Geometry: final body of the model. Coordinates: model frame, mm. Face numbers are marked on the shaded views. Round coordinates to 2 decimals unless told otherwise and drop trailing zeros. Loops run counter-clockwise (first coordinate to the right, second up) from the corner with the lowest first, then second, coordinate; pieces in that order, holes last. Notation, with made-up numbers: (-15.75, -9) -> (33.25, -9) arc R16 cw to (33.25, -5) -> close; hole circle Ø10 at (15.5, 9). An arc over 180 degrees is marked (long way). Answer in a Markdown table with one row per item.
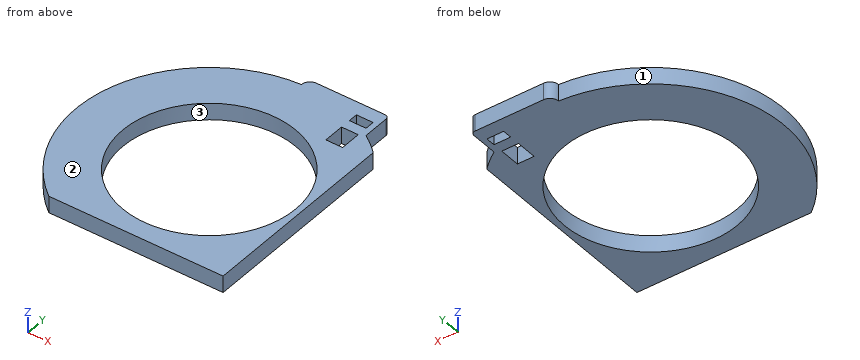
```python
from build123d import *

# Parameters (mm, degrees)
SKETCH1_R           = 25.869040911
BOSS_EXTRUDE1_DEPTH = 5
CUT_EXTRUDE1_REACH  = 7
SKETCH2_W           = 5
SKETCH2_H           = 2.807032228
SKETCH2_H_2         = 6.272905991


with BuildPart() as part:
    # Sketch1 → Boss-Extrude1 (new body)
    with BuildSketch(Plane.XY):
        with BuildLine():
            Line((27.585503877, -31.392941885), (-24.576892053, -31.392941885))
            ThreePointArc((-24.576892053, -31.392941885), (-38.026656197, 11.979726275), (-2.145068244, 39.811293691))
            ThreePointArc((-2.145068244, 39.811293691), (-1.391692185, 41.630104391), (0.427118514, 42.38348045))
            Line((0.427118514, 42.38348045), (20.910674351, 42.38348045))
            ThreePointArc((20.910674351, 42.38348045), (21.815017729, 42.008889157), (22.189609022, 41.104545778))
            Line((22.189609022, 41.104545778), (22.189609022, 33.1234309))
            ThreePointArc((22.189609022, 33.1234309), (24.981909543, 31.071604702), (27.585503877, 28.785072503))
            Line((27.585503877, 28.785072503), (27.585503877, -31.392941885))
        make_face()
        Circle(SKETCH1_R, mode=Mode.SUBTRACT)
    extrude(amount=BOSS_EXTRUDE1_DEPTH)

    # Sketch2 → Cut-Extrude1 (cut, up to next)
    with BuildSketch(Plane(origin=(0, 0, 0), x_dir=(-1, 0, 0), z_dir=(0, 0, -1)), mode=Mode.PRIVATE) as cut_extrude1_sk1:
        with Locations((-18, 36.803720292)):
            Rectangle(SKETCH2_W, SKETCH2_H)
    cut_extrude1_tool1 = extrude(cut_extrude1_sk1.sketch, amount=-CUT_EXTRUDE1_REACH, mode=Mode.PRIVATE) & part.part
    add(cut_extrude1_tool1.solids().sort_by_distance((18, 36.80372, 0))[0], mode=Mode.SUBTRACT)
    # Sketch2 → Cut-Extrude1 (cut, up to next)
    with BuildSketch(Plane(origin=(0, 0, 0), x_dir=(-1, 0, 0), z_dir=(0, 0, -1)), mode=Mode.PRIVATE) as cut_extrude1_sk2:
        with Locations((-18, 29.132248973)):
            Rectangle(SKETCH2_W, SKETCH2_H_2)
    cut_extrude1_tool2 = extrude(cut_extrude1_sk2.sketch, amount=-CUT_EXTRUDE1_REACH, mode=Mode.PRIVATE) & part.part
    add(cut_extrude1_tool2.solids().sort_by_distance((18, 29.132249, 0))[0], mode=Mode.SUBTRACT)


solid = part.part
```
Item 1: Section query B-B, the plane z = 2.65. Output: boundary loops of the cut face in (x, y).
Ans:
| item | result |
|---|---|
| outline | (-24.58, -31.39) -> (27.59, -31.39) -> (27.59, 28.79) arc R39.87 ccw to (22.19, 33.12) -> (22.19, 41.1) arc R1.28 ccw to (20.91, 42.38) -> (0.43, 42.38) arc R2.57 ccw to (-2.15, 39.81) arc R39.87 ccw to start; hole circle Ø51.74 at (0, 0); hole (15.5, 26) -> (20.5, 26) -> (20.5, 32.27) -> (15.5, 32.27) -> close; hole (15.5, 35.4) -> (20.5, 35.4) -> (20.5, 38.21) -> (15.5, 38.21) -> close |
Item 2: First-contact query: P1, Ø2, axis at y = 37.5, z = 3, coming from the -X side; P2, Ø1, axis at x = -25.5, z = 3, coming from the -Y side; P3, Ø2.5, axis at y = 36.5, z = 3, coming from the +X side. Flat tips, straight axial feed; report the tip coordinate or a pass-through.
Ans:
| item | result |
|---|---|
| P1 | x = -16.04 |
| P2 | y = -31.06 |
| P3 | x = 22.19 |
Item 3: Section query C-C, the plane x = 12. Output: boundary loops of the cut face in (y, z), and give its area (3 significant figures).
Ans:
| item | result |
|---|---|
| outline | (-31.39, 0) -> (-22.92, 0) -> (-22.92, 5) -> (-31.39, 5) -> close; (22.92, 0) -> (42.38, 0) -> (42.38, 5) -> (22.92, 5) -> close |
| area | 140 mm2 |
Item 4: Ray query, L1, parallel to Y at x = 20, z = 2.7; L2, parallel to Y at x = 17.5, z = 3.1; L3, parallel to Y at x = 0, z = 3.65. Return the intervals inside material, ascending.
Ans:
| item | result |
|---|---|
| L1 | -31.39 to -16.41, 16.41 to 26, 32.27 to 35.4, 38.21 to 42.38 |
| L2 | -31.39 to -19.05, 19.05 to 26, 32.27 to 35.4, 38.21 to 42.38 |
| L3 | -31.39 to -25.87, 25.87 to 42.35 |
Item 5: Mould query, pull axis X, two halves, no side actions, for the marked faces 1, 2 and 3. Classes: released by +X, released by -X, zero draft, split by the parting line, or undercut.
Ans:
| item | result |
|---|---|
| face 1 | released by -X |
| face 2 | zero draft |
| face 3 | undercut |
Item 6: Section query A-A, the plane y = 0. Output: boundary loops of the cut face in (x, z).
Ans:
| item | result |
|---|---|
| outline | (-39.87, 0) -> (-25.87, 0) -> (-25.87, 5) -> (-39.87, 5) -> close; (25.87, 0) -> (27.59, 0) -> (27.59, 5) -> (25.87, 5) -> close |
